Source: CAD feature listing. Evaluate the final solid. Frame: model axes, mm. Face numbers are marked on the shaded views. A direction names the side the tool comes from. Give positions to 0.01 mm unless a question says otherwise; leave off trailing zeros. Order: outer loops, then holes, each group sorted by start corner. A loop starts at its lowest first (then second) coordinate and runs counter-clockwise, first axis right, second up. Notation, with made-up numbers: M 22,69.25 L 29,69.25 A3 cw 29,74.25 Z; hole C 82.25,7 d9. An arc over 180 degrees is marked long. Answer as a JSON object with one key per item and string values. Group by question number.
1. Section query D-D (x = 26.5). Output: boundary loops of the cut face in (y, z).
2. Section query C-C (z = 10). Output: boundary loops of the cut face in (x, y).
3. Pin query (flat end, axial travel): P1, Ø9, axis at x = 13.5, y = 18, coming from the +Z side; P2, Ø9, axis at x = 14.5, y = 15.5, coming from the -Z side. Return the tip coordinate at first contact, or that it passes through.
4. Section query A-A (y = 17.5). Output: boundary loops of the cut face in (x, z), plus the area to 3 significant figures.
5. Set-up query: the marked faces 1, 2 and 3. Return all of +Z, -Z, +X, -X, +Y, -Y with unobstructed straight access to the full face (end or side cutting, diameter ignored); none if empty.
6. Section query B-B (y = 9). Output: boundary loops of the cut face in (x, z), plus the area to 3 significant figures.
7. Material intervals for L1, parallel to Z at x = 19.5, y = 8; L2, parallel to X at y = 26, z = 11, sorted ascending. Write a range as [from, to].
from build123d import *

# Parameters (mm, degrees)
SKETCH_1_W      = 60
SKETCH_1_H      = 40
EXTRUDE_1_DEPTH = 6
SKETCH_2_W      = 40
SKETCH_2_H      = 36
EXTRUDE_2_DEPTH = 6
EXTRUDE_START   = -2
EXTRUDE_3_DEPTH = 4


# Read off the part's stored shape, not the designer's step: 凸台-拉伸3
with BuildPart() as part:
    # 草图1 → 凸台-拉伸1 (new body)
    with BuildSketch(Plane(origin=(0, 0, 0), x_dir=(1, 0, 0), z_dir=(0, 1, 0))):
        with Locations((30, 0)):
            Rectangle(SKETCH_1_W, SKETCH_1_H)
    extrude(amount=EXTRUDE_1_DEPTH)

    # 草图2 → 凸台-拉伸2 (add)
    with BuildSketch(Plane(origin=(0, 0, 0), x_dir=(0, 0, -1), z_dir=(1, 0, 0))):
        with Locations((0, 18)):
            Rectangle(SKETCH_2_W, SKETCH_2_H)
    extrude(amount=EXTRUDE_2_DEPTH)

    # 凸台-拉伸3 outline → 凸台-拉伸3 (add)
    with BuildSketch(Plane.XY.offset(EXTRUDE_START)):
        Polygon((24, 6), (6, 24), (6, 6), align=None)
    extrude(amount=EXTRUDE_3_DEPTH)


solid = part.part
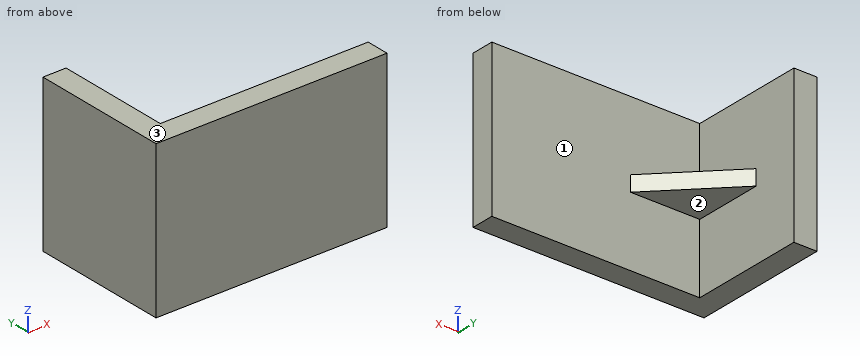
Answer sheet:
{
 "1": {"outline": "M 0,-20 L 6,-20 L 6,20 L 0,20 Z"},
 "2": {"outline": "M 0,0 L 60,0 L 60,6 L 6,6 L 6,36 L 0,36 Z"},
 "3": {"P1": "z = 2", "P2": "z = -2"},
 "4": {"outline": "M 0,-20 L 6,-20 L 6,-2 L 12.5,-2 L 12.5,2 L 6,2 L 6,20 L 0,20 Z", "area": "266 mm^2"},
 "5": {"face 1": "+X, +Y", "face 2": "-Z, +X, +Y", "face 3": "+Z, +X, -X, +Y, -Y"},
 "6": {"outline": "M 0,-20 L 6,-20 L 6,-2 L 21,-2 L 21,2 L 6,2 L 6,20 L 0,20 Z", "area": "300 mm^2"},
 "7": {"L1": "[-2, 2]", "L2": "[0, 6]"}
}
